Geometry check sheet. Reference: the model listing, model coordinates, mm. Face numbers are marked on the shaded views. Round coordinates to 2 decimals unless told otherwise and drop trailing zeros. Write each loop counter-clockwise with the first axis right and the second up, starting at its lowest first coordinate (ties: lowest second). Pieces come first, ordered by that corner, then holes. Notation, with made-up numbers: (77.5, 55.25) -> (85.5, 55.25) arc R16 cw to (85.5, 80.25) -> close; hole circle Ø2 at (49.25, -26.5). An arc over 180 degrees is marked (long way). Return JSON: item names as keys, results as strings. Group by question number.
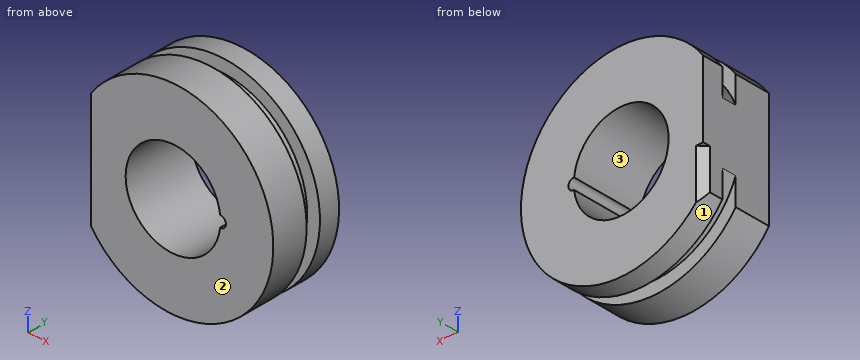
from build123d import *

# Parameters (mm, degrees)
EXTRUDE_1_DEPTH     = 19.75
SKETCH_2_R          = 13
CUT_EXTRUDE_2_DEPTH = 20.75
SKETCH_3_W          = 5
SKETCH_3_H          = 4
SKETCH_4_R          = 1.5
CUT_EXTRUDE_3_DEPTH = 20.75
CUT_EXTRUDE_4_DEPTH = 23.69


with BuildPart() as part:
    # Эскиз1 → Бобышка-Вытянуть1 (new body)
    with BuildSketch(Plane(origin=(0, 0, 0), x_dir=(1, 0, 0), z_dir=(0, 1, 0))):
        with BuildLine():
            Line((-22.5, 15.811388301), (-22.5, -15.811388301))
            ThreePointArc((-22.5, -15.811388301), (27.5, 0), (-22.5, 15.811388301))
        make_face()
    extrude(amount=EXTRUDE_1_DEPTH)

    # Эскиз2 → Вырез-Вытянуть2 (cut, through all)
    with BuildSketch(Plane(origin=(0, 0, 0), x_dir=(1, 0, 0), z_dir=(0, 1, 0))):
        Circle(SKETCH_2_R)
    extrude(amount=CUT_EXTRUDE_2_DEPTH, mode=Mode.SUBTRACT)

    # Эскиз3 → Вырез-Повернуть1 (revolve, cut)
    with BuildSketch(Plane(origin=(0, 0, 0), x_dir=(0, 0, -1), z_dir=(1, 0, 0))):
        with Locations((-26.5, 12)):
            Rectangle(SKETCH_3_W, SKETCH_3_H)
    revolve(axis=Axis((0, 0, 0), (0, 1, 0)), mode=Mode.SUBTRACT)

    # Эскиз4 → Вырез-Вытянуть3 (cut, through all)
    with BuildSketch(Plane(origin=(0, 0, 0), x_dir=(1, 0, 0), z_dir=(0, 1, 0))):
        with Locations((13, 0)):
            Circle(SKETCH_4_R)
    extrude(amount=CUT_EXTRUDE_3_DEPTH, mode=Mode.SUBTRACT)

    # Эскиз5 → Вырез-Вытянуть4 (cut, through all)
    with BuildSketch(Plane.XY.offset(-4.81)):
        Polygon((-22.5, 19.75), (-20.5, 19.75), (-22.5, 17.75), align=None)
    extrude(amount=-CUT_EXTRUDE_4_DEPTH, mode=Mode.SUBTRACT)


solid = part.part
1) Sectioned sample at B-B on x = 0. Enter the section's corners in (y, z).
2) Sectioned sample at D-D on y = 11.5. Enter the section's corners in (x, z), and give its area (3 significant figures).
3) Mould release check, pull along Z, two halves, no side actions. Record for the marked faces 1, 2 and 3: +Z half, -Z half, draft (parallel to the pull), parting line (faces both ways), or undercut.
4) Sectioned sample at A-A on z = 0. Enter the section's corners in (x, y).
5) Go/stop test with flat-tipped pins: P1, Ø6, axis at x = -8, y = 16, coming from the -Z side; P2, Ø5, axis at x = -5, y = 11, coming from the -Z side; P3, Ø8, axis at x = 8, z = -1, coming from the -Y side; P4, Ø8, axis at x = 10, y = 6.5, coming from the -Z side. Record where each tip stops, or that it passes through.
6) Material ranges on probe 1 along Y at (x, z) = (0, -25); probe 2 along X at (y, z) = (13.5, 0); probe 3 along X at (y, z) = (4.5, 0), recorded low to high. Write a range as [from, to].
7) Sectioned sample at C-C on x = -10. Enter the section's corners in (y, z).
Evaluation:
{
 "1": {"outline": "(0, -27.5) -> (10, -27.5) -> (10, -24) -> (14, -24) -> (14, -27.5) -> (19.75, -27.5) -> (19.75, -13) -> (0, -13) -> close; (0, 13) -> (19.75, 13) -> (19.75, 27.5) -> (14, 27.5) -> (14, 24) -> (10, 24) -> (10, 27.5) -> (0, 27.5) -> close"},
 "2": {"outline": "(-22.5, -8.35) arc R24 ccw (long way) to (-22.5, 8.35) -> close; hole (12.91, -1.5) arc R1.5 ccw (long way) to (12.91, 1.5) arc R13 ccw (long way) to start", "area": "1,260 mm2"},
 "3": {"face 1": "parting line", "face 2": "draft", "face 3": "undercut"},
 "4": {"outline": "(-22.5, 0) -> (-13, 0) -> (-13, 19.75) -> (-22.5, 19.75) -> close; (14.5, 0) -> (27.5, 0) -> (27.5, 10) -> (24, 10) -> (24, 14) -> (27.5, 14) -> (27.5, 19.75) -> (14.5, 19.75) -> close"},
 "5": {"P1": "stops at z = -27.04", "P2": "stops at z = -27.37", "P3": "passes through", "P4": "stops at z = -26.84"},
 "6": {"probe 1": "y = [0, 10], [14, 19.75]", "probe 2": "x = [-22.5, -13], [14.5, 24]", "probe 3": "x = [-22.5, -13], [14.5, 27.5]"},
 "7": {"outline": "(0, -25.62) -> (10, -25.62) -> (10, -21.82) -> (14, -21.82) -> (14, -25.62) -> (19.75, -25.62) -> (19.75, -8.31) -> (0, -8.31) -> close; (0, 8.31) -> (19.75, 8.31) -> (19.75, 25.62) -> (14, 25.62) -> (14, 21.82) -> (10, 21.82) -> (10, 25.62) -> (0, 25.62) -> close"}
}
